Here's how the part is built. I have some questions about the finished solid (model axes, mm). A direction names the side the tool comes from. Give positions to 0.01 mm unless a question says otherwise; leave off trailing zeros. Order: outer loops, then holes, each group sorted by start corner. A loop starts at its lowest first (then second) coordinate and runs counter-clockwise, first axis right, second up. Notation, with made-up numbers: (-31.5, -24.5) -> (-21.5, -24.5) arc R10 ccw to (-21.5, -6.5) -> close; hole circle Ø3 at (-29, 33). An arc over 180 degrees is marked (long way). Write each question's results on one line, items separated by ' | '. Start each with the question number.
Q1. Imagine slicing it at C-C, the plane x = 1.5. Please give me the cut outline in (y, z), then the cut area to 3 significant figures.
Q2. I need wall thicknesses on line 1 along X through (y, z) = (-24.5, 6.5); line 2 along Y through (x, z) = (-49, 5) (3 decimals); line 3 along Y through (x, z) = (-41, 1.35). Which ranges of each line are inside material? Lowest first, please. Write a range as [from, to].
Q3. For faces 1 (the face through (37.93, -12.22, 4.44)), 2 (the face through (-36, 0, 1)), which set-ups out of +Z, -Z, +X, -X, +Y, -Y let a thin tool reach every point of the face, with its end or its side?
Q4. Thinking about a two-plate mould opening in Y: for faces 3 (the face through (60, -1, 4)), 4 (the face through (50.5, -41.8, 4.4)), 5 (the face through (1, 50, 4)), which applies, pulls with the +Y half, pulls with the -Y half, needs draft (parallel to the pull), parting line crosses it, or undercut?
Q5. I'm going to push flat-ended pins straight in: pin 1 (4 mm diameter, centred on x = 49, y = 39, fed in from -Z); pin 2 (6 mm diameter, centred on x = 41, y = 0, fed in from -Z). Where does each tip first touch, or does it pass through?
Q6. Imagine slicing it at B-B, the plane y = -22.5. Please give me the cut outline in (x, z).
Q7. Imagine slicing it at A-A, the plane x = -41. Please give me the cut outline in (y, z).
```python
from build123d import *

# Parameters (mm, degrees)
F0_R     = 3.175
F1_DEPTH = 9
F2_DEPTH = 3
F4_R     = 0.5


with BuildPart() as f1:
    # F0 (on Top) → F1 (new body)
    with BuildSketch(Plane.XY):
        with BuildLine():
            Line((0, 17.5), (0, 50))
            Line((0, 50), (-60, 50))
            Line((-60, 50), (-60, 0))
            Line((-60, 0), (-46, 0))
            ThreePointArc((-46, 0), (-41, 5), (-36, 0))
            Line((-36, 0), (-17.5, 0))
            ThreePointArc((-17.5, 0), (-12.3743686708, 12.3743686708), (0, 17.5))
        make_face()
        with Locations((-45.768439, 22.5)):
            Circle(F0_R, mode=Mode.SUBTRACT)
        with Locations((-49, 39)):
            Circle(F0_R, mode=Mode.SUBTRACT)
        with BuildLine():
            Line((60, 50), (0, 50))
            Line((0, 50), (0, 17.5))
            ThreePointArc((0, 17.5), (12.3743686708, 12.3743686708), (17.5, 0))
            Line((17.5, 0), (36, 0))
            ThreePointArc((36, 0), (41, 5), (46, 0))
            Line((46, 0), (60, 0))
            Line((60, 0), (60, 50))
        make_face()
        with Locations((45.768439, 22.5)):
            Circle(F0_R, mode=Mode.SUBTRACT)
        with Locations((49, 39)):
            Circle(F0_R, mode=Mode.SUBTRACT)
        with BuildLine():
            Line((36, 0), (17.5, 0))
            ThreePointArc((17.5, 0), (12.3743686708, -12.3743686708), (0, -17.5))
            Line((0, -17.5), (0, -50))
            Line((0, -50), (60, -50))
            Line((60, -50), (60, 0))
            Line((60, 0), (46, 0))
            ThreePointArc((46, 0), (44.2486753365, -3.8008036726), (40.2215565768, -4.9390308601))
            ThreePointArc((40.2215565768, -4.9390308601), (42.2722916819, -7.6662673034), (43, -11))
            ThreePointArc((43, -11), (28.5909784575, -15.7879476676), (37.268889283, -3.3284850635))
            ThreePointArc((37.268889283, -3.3284850635), (36.3279793673, -1.7810736109), (36, 0))
        make_face()
        with Locations((49, -39)):
            Circle(F0_R, mode=Mode.SUBTRACT)
        with Locations((45.768439, -22.5)):
            Circle(F0_R, mode=Mode.SUBTRACT)
        with BuildLine():
            ThreePointArc((0, -17.5), (-12.3743686708, -12.3743686708), (-17.5, 0))
            Line((-17.5, 0), (-36, 0))
            ThreePointArc((-36, 0), (-41, -5), (-46, 0))
            Line((-46, 0), (-60, 0))
            Line((-60, 0), (-60, -50))
            Line((-60, -50), (0, -50))
            Line((0, -50), (0, -17.5))
        make_face()
        with Locations((-49, -39)):
            Circle(F0_R, mode=Mode.SUBTRACT)
        with Locations((-45.768439, -22.5)):
            Circle(F0_R, mode=Mode.SUBTRACT)
        with BuildLine():
            ThreePointArc((40.2215565768, -4.9390308601), (38.6057393466, -4.3894778646), (37.268889283, -3.3284850635))
            ThreePointArc((37.268889283, -3.3284850635), (28.5909784575, -15.7879476676), (43, -11))
            ThreePointArc((43, -11), (42.2722916819, -7.6662673034), (40.2215565768, -4.9390308601))
        make_face()
        with Locations((35, -11)):
            Circle(F0_R, mode=Mode.SUBTRACT)
        with BuildLine():
            Line((38.42, 0), (36, 0))
            ThreePointArc((36, 0), (36.3279793673, -1.7810736109), (37.268889283, -3.3284850635))
            ThreePointArc((37.268889283, -3.3284850635), (38.8308170454, -3.9768354167), (40.2215565768, -4.9390308601))
            ThreePointArc((40.2215565768, -4.9390308601), (44.2486753365, -3.8008036726), (46, 0))
            Line((46, 0), (43.58, 0))
            ThreePointArc((43.58, 0), (41, -2.58), (38.42, 0))
        make_face()
        with BuildLine():
            ThreePointArc((46, 0), (41, 5), (36, 0))
            Line((36, 0), (38.42, 0))
            ThreePointArc((38.42, 0), (41, 2.58), (43.58, 0))
            Line((43.58, 0), (46, 0))
        make_face()
        with BuildLine():
            Line((-38.42, 0), (-36, 0))
            ThreePointArc((-36, 0), (-41, 5), (-46, 0))
            Line((-46, 0), (-43.58, 0))
            ThreePointArc((-43.58, 0), (-41, 2.58), (-38.42, 0))
        make_face()
        with BuildLine():
            ThreePointArc((-46, 0), (-41, -5), (-36, 0))
            Line((-36, 0), (-38.42, 0))
            ThreePointArc((-38.42, 0), (-41, -2.58), (-43.58, 0))
            Line((-43.58, 0), (-46, 0))
        make_face()
        with BuildLine():
            ThreePointArc((40.2215565768, -4.9390308601), (38.8308170454, -3.9768354167), (37.268889283, -3.3284850635))
            ThreePointArc((37.268889283, -3.3284850635), (38.6057393466, -4.3894778646), (40.2215565768, -4.9390308601))
        make_face()
        with BuildLine():
            Line((0, 6), (0, 17.5))
            ThreePointArc((0, 17.5), (-12.3743686708, 12.3743686708), (-17.5, 0))
            Line((-17.5, 0), (-6, 0))
            ThreePointArc((-6, 0), (-4.2426406871, 4.2426406871), (0, 6))
        make_face()
        with BuildLine():
            ThreePointArc((17.5, 0), (12.3743686708, 12.3743686708), (0, 17.5))
            Line((0, 17.5), (0, 6))
            ThreePointArc((0, 6), (4.2426406871, 4.2426406871), (6, 0))
            Line((6, 0), (17.5, 0))
        make_face()
        with BuildLine():
            ThreePointArc((0, -17.5), (12.3743686708, -12.3743686708), (17.5, 0))
            Line((17.5, 0), (6, 0))
            ThreePointArc((6, 0), (4.2426406871, -4.2426406871), (0, -6))
            Line((0, -6), (0, -17.5))
        make_face()
        with BuildLine():
            Line((-6, 0), (-17.5, 0))
            ThreePointArc((-17.5, 0), (-12.3743686708, -12.3743686708), (0, -17.5))
            Line((0, -17.5), (0, -6))
            ThreePointArc((0, -6), (-4.2426406871, -4.2426406871), (-6, 0))
        make_face()
    extrude(amount=F1_DEPTH)


with BuildPart() as f2:
    # F0 (on Top) → F2 (new body)
    with BuildSketch(Plane.XY):
        with BuildLine():
            Line((38.42, 0), (36, 0))
            ThreePointArc((36, 0), (36.3279793673, -1.7810736109), (37.268889283, -3.3284850635))
            ThreePointArc((37.268889283, -3.3284850635), (38.8308170454, -3.9768354167), (40.2215565768, -4.9390308601))
            ThreePointArc((40.2215565768, -4.9390308601), (44.2486753365, -3.8008036726), (46, 0))
            Line((46, 0), (43.58, 0))
            ThreePointArc((43.58, 0), (41, -2.58), (38.42, 0))
        make_face()
        with BuildLine():
            ThreePointArc((46, 0), (41, 5), (36, 0))
            Line((36, 0), (38.42, 0))
            ThreePointArc((38.42, 0), (41, 2.58), (43.58, 0))
            Line((43.58, 0), (46, 0))
        make_face()
        with BuildLine():
            ThreePointArc((40.2215565768, -4.9390308601), (38.8308170454, -3.9768354167), (37.268889283, -3.3284850635))
            ThreePointArc((37.268889283, -3.3284850635), (38.6057393466, -4.3894778646), (40.2215565768, -4.9390308601))
        make_face()
    extrude(amount=F2_DEPTH)


with BuildPart() as f2b:
    # F0 (on Top) → F2, piece 2 (new body)
    with BuildSketch(Plane.XY):
        with BuildLine():
            Line((-38.42, 0), (-36, 0))
            ThreePointArc((-36, 0), (-41, 5), (-46, 0))
            Line((-46, 0), (-43.58, 0))
            ThreePointArc((-43.58, 0), (-41, 2.58), (-38.42, 0))
        make_face()
        with BuildLine():
            ThreePointArc((-46, 0), (-41, -5), (-36, 0))
            Line((-36, 0), (-38.42, 0))
            ThreePointArc((-38.42, 0), (-41, -2.58), (-43.58, 0))
            Line((-43.58, 0), (-46, 0))
        make_face()
    extrude(amount=F2_DEPTH)


with BuildPart() as f1_1:
    add(f1.part)

    # F3: cut F2b, F2
    add(f2b.part, mode=Mode.SUBTRACT)
    add(f2.part, mode=Mode.SUBTRACT)

    # F4
    f4_edges = [f1_1.edges().sort_by_distance(p)[0] for p in [
        (60, 50, 4.5),
        (60, -50, 4.5),
        (-60, 50, 4.5),
        (-60, -50, 4.5),
    ]]
    fillet(f4_edges, radius=F4_R)


solid = f1_1.part
```
Geometry check:
1) outline: (-50, 0) -> (-5.81, 0) -> (-5.81, 9) -> (-50, 9) -> close; (5.81, 0) -> (50, 0) -> (50, 9) -> (5.81, 9) -> close | area: 795 mm²
2) line 1: [-60, -48.23], [-43.3, 43.3], [48.23, 60] | line 2: [-50, -42.175], [-35.825, 35.825], [42.175, 50] | line 3: [-50, -5], [5, 50]
3) face 1: +Z, -Z | face 2: -Z
4) face 3: needs draft | face 4: undercut | face 5: pulls with the +Y half
5) pin 1: through | pin 2: z = 3
6) outline: (-60, 0) -> (-48.94, 0) -> (-48.94, 9) -> (-60, 9) -> close; (-42.59, 0) -> (42.59, 0) -> (42.59, 9) -> (-42.59, 9) -> close; (48.94, 0) -> (60, 0) -> (60, 9) -> (48.94, 9) -> close
7) outline: (-50, 0) -> (-5, 0) -> (-5, 3) -> (-2.58, 3) -> (-2.58, 9) -> (-50, 9) -> close; (2.58, 3) -> (5, 3) -> (5, 0) -> (50, 0) -> (50, 9) -> (2.58, 9) -> close
